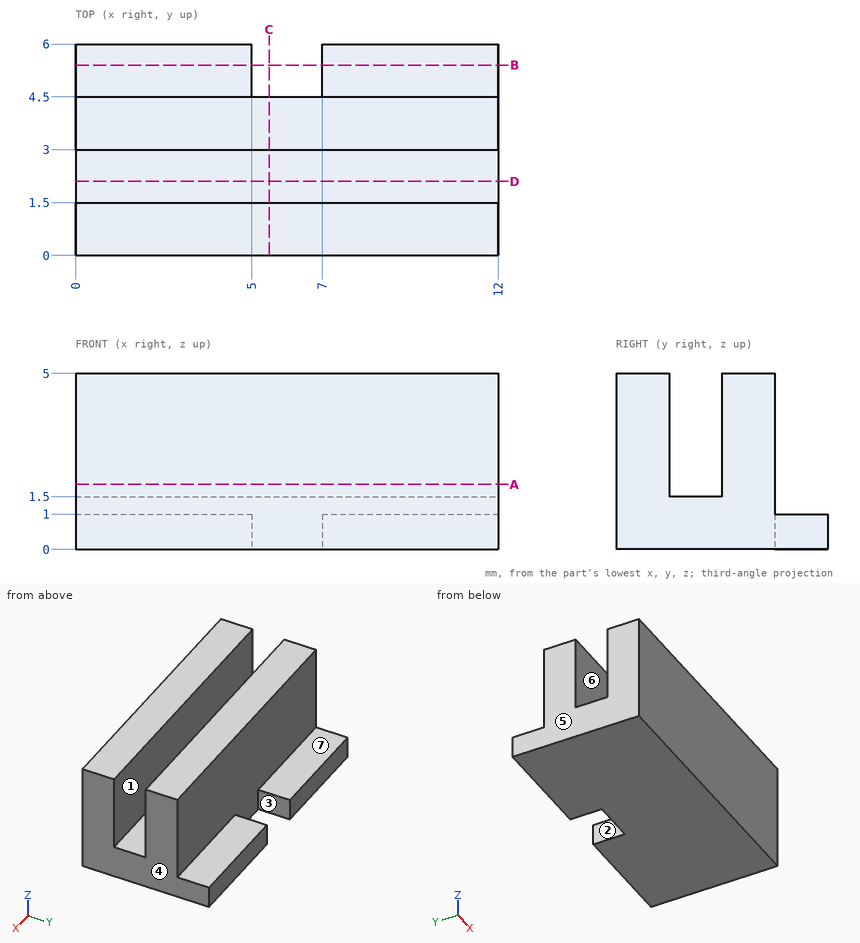
Source: three-view drawing plus pictorial views. Frame: mm from the lowest corner of the part. A direction names the side the tool comes from. Give positions to 0.01 mm unless a question says otherwise; leave off trailing zeros. Loops run counter-clockwise (first coordinate to the right, second up) from the corner with the lowest first, then second, coordinate; pieces in that order, holes last. Notation, with made-up numbers: (-1, 44.25) -> (46, 44.25) arc R20 ccw to (46, 57.25) -> close; hole circle Ø8 at (-3, 46.25). An arc over 180 degrees is marked (long way). Use a Markdown table: item, result. Add a question column.
(1) Pull-direction query (X, two-part tool) for the marked faces 1, 2, 3 and 4; classes: +X half, -X half, draft (parallel to the pull), parting line (faces both ways), or undercut.
(2) Section query A-A (z = 1.85). Output: boundary loops of the cut face in (x, y), then the cut area to 3 significant figures.
(3) Section query C-C (x = 5.5). Output: boundary loops of the cut face in (y, z).
(4) First-contact query: pin 1 Ø0.8 at (x, y) = (2.5, 5.5) entering from +Z; pin 2 Ø1 at (x, z) = (5.5, 3) entering from +Y. Flat tips, straight axial feed; report the tip coordinate or a pass-through.
(5) Ray query, line 1 (Y direction, x = 5, z = 2.9); line 2 (Z direction, x = 1, y = 2.1); line 3 (Y direction, x = 6.75, z = 0.75). Return the intervals inside material, ascending.
(6) Section query B-B (y = 5.4). Output: boundary loops of the cut face in (x, z).
(7) Section query D-D (y = 2.1). Output: boundary loops of the cut face in (x, z), then the cut area to 3 significant figures.
(8) Access query for the marked faces 5, 6 and 7. Directions: +Z, -Z, +X, -X, +Y, -Y. A direction counts if a zero-diameter tool reaches every point of the face in a straight line with its end or side. Return the directions, or none.
Checked values:
| question | item | result |
|---|---|---|
| 1 | face 1 | draft |
| 1 | face 2 | undercut |
| 1 | face 3 | undercut |
| 1 | face 4 | +X half |
| 2 | outline | (0, 0) -> (12, 0) -> (12, 1.5) -> (0, 1.5) -> close; (0, 3) -> (12, 3) -> (12, 4.5) -> (0, 4.5) -> close |
| 2 | area | 36.0 mm^2 |
| 3 | outline | (0, 0) -> (4.5, 0) -> (4.5, 5) -> (3, 5) -> (3, 1.5) -> (1.5, 1.5) -> (1.5, 5) -> (0, 5) -> close |
| 4 | pin 1 | z = 1 |
| 4 | pin 2 | y = 4.5 |
| 5 | line 1 | 0 to 1.5, 3 to 4.5 |
| 5 | line 2 | 0 to 1.5 |
| 5 | line 3 | 0 to 4.5 |
| 6 | outline | (0, 0) -> (5, 0) -> (5, 1) -> (0, 1) -> close; (7, 0) -> (12, 0) -> (12, 1) -> (7, 1) -> close |
| 7 | outline | (0, 0) -> (12, 0) -> (12, 1.5) -> (0, 1.5) -> close |
| 7 | area | 18.0 mm^2 |
| 8 | face 5 | +Z, -Z, -X, +Y, -Y |
| 8 | face 6 | +Z, +X, -X |
| 8 | face 7 | +Z, +X, -X, +Y |
